Build history of the part. All positions in model axes, mm. Give positions to 0.01 mm unless a question says otherwise; leave off trailing zeros. Order: outer loops, then holes, each group sorted by start corner. A loop starts at its lowest first (then second) coordinate and runs counter-clockwise, first axis right, second up. Notation, with made-up numbers: (58, 31) - (93, 31) arc R21 ccw to (93, 61) - close; hole circle Ø3 at (-5, 71.5). An arc over 180 degrees is marked (long way). Write each question's results on one line, items separated by ' | '. Start each with the question number.
from build123d import *

# Parameters (mm, degrees)
SKETCH1_W           = 135
SKETCH1_H           = 38.1
SKETCH1_R           = 1.15
SKETCH1_R_2         = 10
BOSS_EXTRUDE1_DEPTH = 2.9718
SKETCH2_R           = 1.5
CUT_EXTRUDE1_DEPTH  = 141.304816721


with BuildPart() as part:
    # Sketch1 → Boss-Extrude1 (new body)
    with BuildSketch(Plane(origin=(0, 0, 0), x_dir=(1, 0, 0), z_dir=(0, 1, 0))):
        with Locations((67.5, 19.05)):
            Rectangle(SKETCH1_W, SKETCH1_H)
        with Locations(Location((80, 8.5718, 0), (0, 0, 270))):
            Circle(SKETCH1_R, mode=Mode.SUBTRACT)
        with Locations(Location((80, 25.5718, 0), (0, 0, 270))):
            Circle(SKETCH1_R, mode=Mode.SUBTRACT)
        with Locations(Location((100, 17.0718, 0), (0, 0, 270))):
            Circle(SKETCH1_R_2, mode=Mode.SUBTRACT)
    extrude(amount=BOSS_EXTRUDE1_DEPTH)

    # Sketch2 → Cut-Extrude1 (cut, through all)
    with BuildSketch(Plane(origin=(0, 2.9718, 0), x_dir=(1, 0, 0), z_dir=(0, 1, 0))):
        with Locations(Location((128, 8.5718, 0), (0, 0, 270))):
            Circle(SKETCH2_R)
        with Locations(Location((7, 8.5718, 0), (0, 0, 270))):
            Circle(SKETCH2_R)
    extrude(amount=-CUT_EXTRUDE1_DEPTH, mode=Mode.SUBTRACT)


solid = part.part
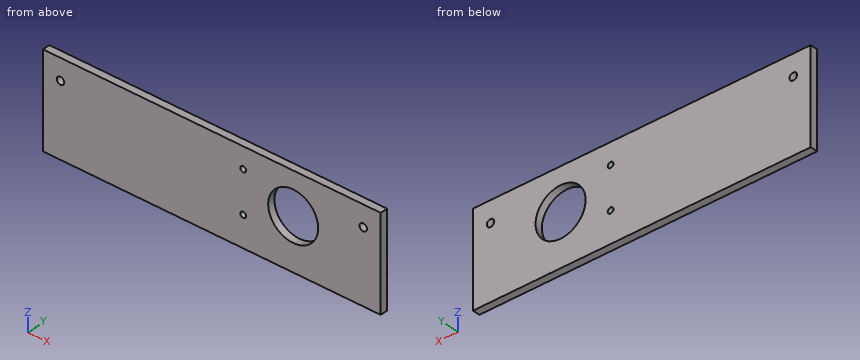
Item 1: Probe line 1 along Z through (x, y) = (80, 1.7); line 2 along X through (y, z) = (0.9, -9); line 3 along X through (y, z) = (1.6, -25). List the from-to ranges inside material, lowest first. Write a range as from..to.
Item 2: Cut at B-B, the plane y = 0.9. List the corners of the cut face in (x, z), then the cut area to 3 significant figures.
Item 3: Cut at A-A, the plane x = 100. List the corners of the cut face in (y, z).
Item 4: Cut at D-D, the plane x = 80. List the corners of the cut face in (y, z).
Item 5: Cut at C-C, the plane z = -22.5. List the corners of the cut face in (x, y).
Values found:
1) line 1: z = -38.1..-26.72, -24.42..-9.72, -7.42..0 | line 2: x = 0..5.56, 8.44..78.93, 81.07..94.1, 105.9..126.56, 129.44..135 | line 3: x = 0..79, 81..93.91, 106.09..135
2) outline: (0, -38.1) - (135, -38.1) - (135, 0) - (0, 0) - close; hole circle Ø3 at (7, -8.57); hole circle Ø2.3 at (80, -25.57); hole circle Ø2.3 at (80, -8.57); hole circle Ø20 at (100, -17.07); hole circle Ø3 at (128, -8.57) | area: 4,810 mm2
3) outline: (0, -38.1) - (2.97, -38.1) - (2.97, -27.07) - (0, -27.07) - close; (0, -7.07) - (2.97, -7.07) - (2.97, 0) - (0, 0) - close
4) outline: (0, -38.1) - (2.97, -38.1) - (2.97, -26.72) - (0, -26.72) - close; (0, -24.42) - (2.97, -24.42) - (2.97, -9.72) - (0, -9.72) - close; (0, -7.42) - (2.97, -7.42) - (2.97, 0) - (0, 0) - close
5) outline: (0, 0) - (91.6, 0) - (91.6, 2.97) - (0, 2.97) - close; (108.4, 0) - (135, 0) - (135, 2.97) - (108.4, 2.97) - close
